Part model, mm, in its own coordinate system. Face numbers are marked on the shaded views. A direction names the side the tool comes from. Give positions to 0.01 mm unless a question says otherwise; leave off trailing zeros. Loops run counter-clockwise (first coordinate to the right, second up) from the corner with the lowest first, then second, coordinate; pieces in that order, holes last. Notation, with made-up numbers: M -5,65.25 L 42,65.25 A24 ccw 42,77.25 Z; hole C 28,64.5 d10. An arc over 180 degrees is marked long. Answer in a Markdown table with one row per item.
Autodesk Inventor part; units mm, degrees
ref_plane "YZ Plane" through (0, 0, 0) normal (1, 0, 0) x (0, 1, 0)
ref_plane "XZ Plane" through (0, 0, 0) normal (0, 1, 0) x (-1, 0, 0)
ref_plane "XY Plane" through (0, 0, 0) normal (0, 0, 1) x (1, 0, 0)
sketch "Sketch1" plane through (0, 0, 0) normal (0, 1, 0) x (-1, 0, 0)
  line L0 (0, 0) -> (42, 0)
  line L1 (42, 0) -> (42, -42)
  line L2 (42, -42) -> (0, -42)
  line L3 (0, -42) -> (0, 0)
  dimension "d0" = 42
  dimension "d1" = 42
extrude "Extrusion1" add sketch "Sketch1" along normal blind 10
chamfer "Chamfer1" distance 4 angle 45 4 edges at (0, 5, 0) (0, 5, -42) (-42, 5, -42) (-42, 5, 0)
sketch "Sketch2" plane through (0, 10, 0) normal (0, 1, 0) x (1, 0, 0)
  point P0 (0, 0)
sketch "Sketch3" plane through (0, 10, 0) normal (0, 1, 0) x (1, 0, 0)
  line L0 (-0.5, 0.5) -> (-41.5, 0.5)
  line L1 (-41.5, 0.5) -> (-41.5, 41.5)
  line L2 (-41.5, 41.5) -> (-0.5, 41.5)
  line L3 (-0.5, 41.5) -> (-0.5, 0.5)
  line L4 (-0.5, 0.5) -> (-41.5, 41.5) construction
  line L5 (-41.5, 0.5) -> (-0.5, 41.5) construction
  point P0 (0, 0)
  point P1 (-21, 21)
  dimension "d7" = 41
  dimension "d8" = 41
extrude "Extrusion2" add sketch "Sketch3" along normal blind 26
fillet "Fillet1" radius 6.35 4 edges at (-41.5, 23, -41.5) (-0.5, 23, -41.5) (-41.5, 23, -0.5) (-0.5, 23, -0.5)
sketch "Sketch4" plane through (0, 36, 0) normal (0, 1, 0) x (1, 0, 0)
  line L0 (0, 0) -> (-42, 0)
  line L1 (-42, 0) -> (-42, 42)
  line L2 (-42, 42) -> (0, 42)
  line L3 (0, 42) -> (0, 0)
  dimension "d12" = 42
  dimension "d13" = 42
extrude "Extrusion3" add sketch "Sketch4" along normal blind 10
chamfer "Chamfer2" distance 4 angle 45 4 edges at (-42, 41, -42) (-42, 41, 0) (0, 41, -42) (0, 41, 0)
sketch "Sketch5" plane through (0, 0, 0) normal (0, -1, 0) x (1, 0, 0)
  circle A0 centre (-21, -21) radius 11
  point P0 (0, 0)
  dimension "d19" = 22
extrude "Extrusion4" add sketch "Sketch5" along normal blind 2
sketch "Sketch6" plane through (-21, -2, -21) normal (0, -1, 0) x (1, 0, 0)
  circle A0 centre (0, 0) radius 2.5
  point P0 (21, 21)
  dimension "d22" = 5
extrude "Extrusion5" add sketch "Sketch6" along normal blind 22
sketch "Sketch7" plane through (0, 0, 0) normal (0, -1, 0) x (1, 0, 0)
  circle A0 centre (-37, -5) radius 1.5
  circle A1 centre (-5, -5) radius 1.5
  circle A2 centre (-5, -37) radius 1.5
  circle A3 centre (-37, -37) radius 1.5
  point P0 (0, 0)
  dimension "d25" = 3
  dimension "d26" = 3
  dimension "d27" = 3
  dimension "d28" = 3
extrude "Extrusion6" cut sketch "Sketch7" against normal blind 3
sketch "Sketch8" plane through (-21, -24, -21) normal (0, -1, 0) x (1, 0, 0)
  circle A0 centre (0, 0) radius 2.5
  arc A1 (-2.2228, 1.1442) -> (2.2228, 1.1442) centre (0, 0) ccw
  line L0 (-2.2228, 1.1442) -> (2.2228, 1.1442)
  point P0 (21, 21)
extrude "Extrusion7" cut sketch "Sketch8" against normal blind 22 contours L0 A0 picked at (0.2976, 1.8759)
properties part number "nema17_84Ncm"
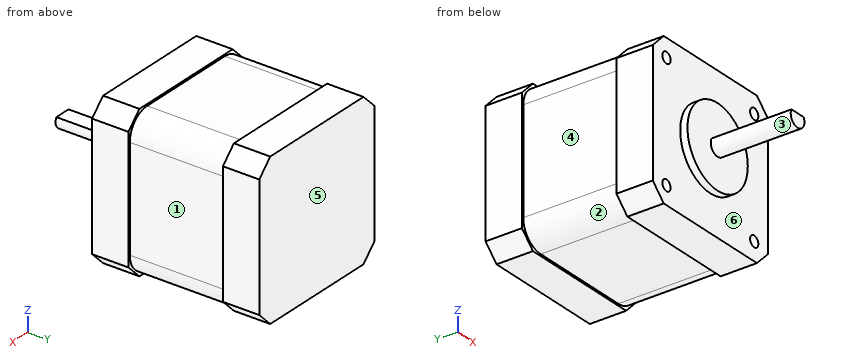
(1) Saw through at D-D (x = -8.5). Write the cut outline in (y, z).
Recorded:
| item | result |
|---|---|
| outline | M 0,-42 L 10,-42 L 10,-41.5 L 36,-41.5 L 36,-42 L 46,-42 L 46,0 L 36,0 L 36,-0.5 L 10,-0.5 L 10,0 L 0,0 Z |
(2) Which spindle directions (+Z, -Z, +X, -X, +Y, -Y) get a long thin tool onto all of the face, cutting with end or side? Do the marked faces 1, 2 and 3. Say none if no direction does.
Recorded:
| item | result |
|---|---|
| face 1 | +Z, -Z, +X |
| face 2 | -Z, -X |
| face 3 | -Y |
(3) Saw through at B-B (y = 11.5). Write the cut outline in (x, z), plus the area to 3 significant figures.
Recorded:
| item | result |
|---|---|
| outline | M -41.5,-35.15 A6.35 ccw -35.15,-41.5 L -6.85,-41.5 A6.35 ccw -0.5,-35.15 L -0.5,-6.85 A6.35 ccw -6.85,-0.5 L -35.15,-0.5 A6.35 ccw -41.5,-6.85 Z |
| area | 1,650 mm^2 |
(4) Drill centre lines: line 1 along Z through (x, y) = (-5, 1); line 2 along X through (y, z) = (31, -26); line 3 along Y through (x, z) = (-12, -33.5). Where is each one in solid material? Low to high.
Recorded:
| item | result |
|---|---|
| line 1 | z = -42 to -38.5, -35.5 to -6.5, -3.5 to 0 |
| line 2 | x = -41.5 to -0.5 |
| line 3 | y = 0 to 46 |
(5) Saw through at A-A (x = -21). Write the cut outline in (y, z).
Recorded:
| item | result |
|---|---|
| outline | M -24,-23.5 L -2,-23.5 L -2,-32 L 0,-32 L 0,-42 L 10,-42 L 10,-41.5 L 36,-41.5 L 36,-42 L 46,-42 L 46,0 L 36,0 L 36,-0.5 L 10,-0.5 L 10,0 L 0,0 L 0,-10 L -2,-10 L -2,-19.86 L -24,-19.86 Z |
(6) Pull direction Y, two halves, no side cores. Call the marked faces 4, 5 and 6: +Y half, -Y half, draft (parallel to the pull), parting line (faces both ways), or undercut.
Recorded:
| item | result |
|---|---|
| face 4 | undercut |
| face 5 | +Y half |
| face 6 | -Y half |
(7) Saw through at C-C (z = -16). Write the cut outline in (x, y), plus the area to 3 significant figures.
Recorded:
| item | result |
|---|---|
| outline | M -42,0 L -30.8,0 L -30.8,-2 L -11.2,-2 L -11.2,0 L 0,0 L 0,10 L -0.5,10 L -0.5,36 L 0,36 L 0,46 L -42,46 L -42,36 L -41.5,36 L -41.5,10 L -42,10 Z |
| area | 1,950 mm^2 |
(8) Pin check, flat tips, straight feed: pin 1 Ø13 at (y, z) = (21.5, -20.5) entering from +X; pin 2 Ø8 at (x, y) = (-18, 21.5) entering from +Z; pin 3 Ø3 at (y, z) = (-5.5, -19.5) entering from +X; pin 4 Ø5 at (y, z) = (-3, -4.5) entering from -X. Stop position of each tip, or through.
Recorded:
| item | result |
|---|---|
| pin 1 | stops at x = -0.5 |
| pin 2 | stops at z = -0.5 |
| pin 3 | stops at x = -18.5 |
| pin 4 | passes through |
